from build123d import *

# Parameters (mm, degrees)
SKETCH1_W           = 3.175
SKETCH1_H           = 25.4
BOSS_EXTRUDE1_DEPTH = 3.175
CUT_EXTRUDE1_DEPTH  = 4.175


with BuildPart() as part:
    # Sketch1 → Boss-Extrude1 (new body)
    with BuildSketch(Plane.XY):
        Polygon((55.5625, -76.2), (74.6125, -76.2), (74.6125, -57.15), (74.6125, -31.75), (74.6125, -12.7), (74.6125, 12.7), (74.6125, 31.75), (74.6125, 57.15), (74.6125, 76.2), (-74.6125, 76.2), (-74.6125, 57.15), (-71.4375, 57.15), (-71.4375, 31.75), (-74.6125, 31.75), (-74.6125, 12.7), (-71.4375, 12.7), (-71.4375, -12.7), (-74.6125, -12.7), (-74.6125, -31.75), (-71.4375, -31.75), (-71.4375, -57.15), (-74.6125, -57.15), (-74.6125, -76.2), (-55.5625, -76.2), (-55.5625, -73.025), (-30.1625, -73.025), (-30.1625, -76.2), (-11.1125, -76.2), (-11.1125, -73.025), (14.2875, -73.025), (14.2875, -76.2), (30.1625, -76.2), (30.1625, -73.025), (55.5625, -73.025), align=None)
        with Locations((76.2, 44.45)):
            Rectangle(SKETCH1_W, SKETCH1_H)
        with Locations((76.2, 0)):
            Rectangle(SKETCH1_W, SKETCH1_H)
        with Locations((76.2, -44.45)):
            Rectangle(SKETCH1_W, SKETCH1_H)
    extrude(amount=BOSS_EXTRUDE1_DEPTH)

    # Sketch2 → Cut-Extrude1 (cut, through all)
    with BuildSketch(Plane.XY.offset(3.175)):
        Polygon((-15.781536726, 38.1), (-38.1, 15.781536726), (-38.1, -15.781536726), (-15.781536726, -38.1), (15.781536726, -38.1), (38.1, -15.781536726), (38.1, 15.781536726), (15.781536726, 38.1), align=None)
    extrude(amount=-CUT_EXTRUDE1_DEPTH, mode=Mode.SUBTRACT)


solid = part.part
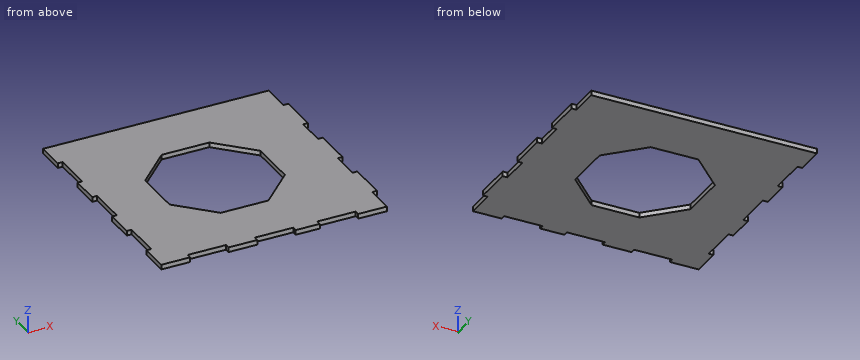
Read the model definition and answer for the solid it produces. Units are mm, in the model's axes. Coordinates: 2 decimals unless noted, no trailing zeros. Loops run counter-clockwise (first coordinate to the right, second up) from the corner with the lowest first, then second, coordinate; pieces in that order, holes last. Notation, with made-up numbers: (-25.5, -18) - (-2.5, -18) arc R25 cw to (-2.5, -3) - close; hole circle Ø1 at (0, -35.5). An arc over 180 degrees is marked (long way). Answer in a Markdown table with one row per item.
Q1. Find section C-C on x = -53. Write down the section's boundary in (y, z) (3 decimals), plus the area to 3 significant figures.
Here are the results:
| item | result |
|---|---|
| outline | (-73.025, 0) - (76.2, 0) - (76.2, 3.175) - (-73.025, 3.175) - close |
| area | 474 mm^2 |
Q2. Straight lines are drawn through the part: line 1 along X through (y, z) = (6.5, 0.9); line 2 along Y through (x, z) = (2.5, 3) (3 decimals); line 3 along X through (y, z) = (-15, 0.9). For each, find the intervals that lie inside material, in ascending order. Write a range as [from, to].
Here are the results:
| item | result |
|---|---|
| line 1 | x = [-71.44, -38.1], [38.1, 77.79] |
| line 2 | y = [-73.025, -38.1], [38.1, 76.2] |
| line 3 | x = [-74.61, -38.1], [38.1, 74.61] |
Q3. Find section B-B on x = 21. Write down the section's boundary in (y, z) (3 decimals), plus the area to 3 significant figures.
Here are the results:
| item | result |
|---|---|
| outline | (-76.2, 0) - (-32.882, 0) - (-32.882, 3.175) - (-76.2, 3.175) - close; (32.882, 0) - (76.2, 0) - (76.2, 3.175) - (32.882, 3.175) - close |
| area | 275 mm^2 |
Q4. Given P1, Ø1.6, axis at y = -20.5, z = 1, coming from the +X side; P2, Ø1, axis at x = 1, z = 2, coming from the -Y side (3 decimals); P3, Ø1, axis at x = 76.5, z = 1.5, coming from the +Y side, each flat-ended and moving along its own axis, determine where each tip first touches the part or whether it passes through.
Here are the results:
| item | result |
|---|---|
| P1 | stops at x = 74.61 |
| P2 | stops at y = -73.025 |
| P3 | stops at y = 57.15 |
Q5. Find section A-A on y = -28.5. Write down the section's boundary in (x, z) (1 decimal).
Here are the results:
| item | result |
|---|---|
| outline | (-74.6, 0) - (-25.4, 0) - (-25.4, 3.2) - (-74.6, 3.2) - close; (25.4, 0) - (74.6, 0) - (74.6, 3.2) - (25.4, 3.2) - close |
Q6. Find section D-D on y = -59. Write down the section's boundary in (x, z) (1 decimal).
Here are the results:
| item | result |
|---|---|
| outline | (-74.6, 0) - (74.6, 0) - (74.6, 3.2) - (-74.6, 3.2) - close |
